from build123d import *

# Parameters (mm, degrees)
EXTRUDE_1_DEPTH     = 15
CUT_EXTRUDE_1_DEPTH = 15
FILLET_1_R          = 1
SKETCH_3_W          = 11.5
SKETCH_3_H          = 1.4
CUT_EXTRUDE_2_DEPTH = 10


with BuildPart() as part:
    # 草图1 → 凸台-拉伸1 (new body)
    with BuildSketch(Plane(origin=(0, 0, 0), x_dir=(1, 0, 0), z_dir=(0, 1, 0))):
        Polygon((-5.74789916, 13.058823529), (2.25210084, 13.058823529), (2.25210084, -11.941176471), (-2.74789916, -11.941176471), (-2.74789916, 4.558823529), (-5.74789916, 4.558823529), align=None)
    extrude(amount=EXTRUDE_1_DEPTH)

    # 草图2 → 切除-拉伸1 (cut)
    with BuildSketch(Plane.ZY.offset(5.74789916)):
        with BuildLine():
            ThreePointArc((-6.483823529, 7.5), (-8.058823529, 9.075), (-9.633823529, 7.5))
            Line((-9.633823529, 7.5), (-6.483823529, 7.5))
        make_face()
        with BuildLine():
            Line((-6.483823529, 7.5), (-9.633823529, 7.5))
            ThreePointArc((-9.633823529, 7.5), (-8.058823529, 5.925), (-6.483823529, 7.5))
        make_face()
    extrude(amount=-CUT_EXTRUDE_1_DEPTH, mode=Mode.SUBTRACT)

    # 圆角1
    fillet_1_edges = [part.edges().sort_by_distance(p)[0] for p in [
        (-2.74789916, 7.5, -4.558823529),
    ]]
    fillet(fillet_1_edges, radius=FILLET_1_R)

    # 草图3 → 切除-拉伸2 (cut)
    with BuildSketch(Plane.ZY.offset(2.74789916)):
        with Locations((1.191176471, 8.2)):
            Rectangle(SKETCH_3_W, SKETCH_3_H)
        with Locations((1.191176471, 6.8)):
            Rectangle(SKETCH_3_W, SKETCH_3_H)
    extrude(amount=-CUT_EXTRUDE_2_DEPTH, mode=Mode.SUBTRACT)


solid = part.part
Model file for the job. Use its own axes, mm. A direction names the side the tool comes from. Give positions to 0.01 mm unless a question says otherwise; leave off trailing zeros. Order: outer loops, then holes, each group sorted by start corner. A loop starts at its lowest first (then second) coordinate and runs counter-clockwise, first axis right, second up. Notation, with made-up numbers: (-33.75, 31) -> (17.25, 31) arc R25 cw to (17.25, 49) -> close; hole circle Ø1 at (24, 82.5). An arc over 180 degrees is marked (long way). Use CSV: the item, a comma, the result in double quotes.
1. Band-saw the part on B-B, the plane y = 7.5. Give the cut face in (x, z), then the cut area to 3 significant figures.
Outcome:
outline,"(-5.75, -13.06) -> (2.25, -13.06) -> (2.25, -9.63) -> (-5.75, -9.63) -> close; (-5.75, -6.48) -> (2.25, -6.48) -> (2.25, -4.56) -> (-2.75, -4.56) -> (-2.75, -3.56) arc R1 cw to (-3.75, -4.56) -> (-5.75, -4.56) -> close; (-2.75, 6.94) -> (2.25, 6.94) -> (2.25, 11.94) -> (-2.75, 11.94) -> close"
area,"68.0 mm²"
2. Band-saw the part on C-C, the plane x = -2. Give the cut face in (y, z) (3 decimals).
Outcome:
outline,"(0, -13.059) -> (15, -13.059) -> (15, 11.941) -> (0, 11.941) -> close; hole circle Ø3.15 at (7.5, -8.059); hole (6.1, -4.559) -> (8.9, -4.559) -> (8.9, 6.941) -> (6.1, 6.941) -> close"
3. Band-saw the part on A-A, the plane z = 5.75. Give the cut face in (x, y), then the cut area to 3 significant figures.
Outcome:
outline,"(-2.75, 0) -> (2.25, 0) -> (2.25, 6.1) -> (-2.75, 6.1) -> close; (-2.75, 8.9) -> (2.25, 8.9) -> (2.25, 15) -> (-2.75, 15) -> close"
area,"61.0 mm²"
4. 3-axis set-ups, long thin cutter, end or side, ignore diameter. For faces 4 (the flat face through (0, 8, -4.559)), 5 (the flat face through (-2.748, 9.1, 4.3)), 6 (the flat face through (0, 7, 6.941)): which of +Z, -Z, +X, -X, +Y, -Y reach the whole face in a straight line?
Outcome:
face 4,"+X"
face 5,"+Z, -X, +Y, -Y"
face 6,"+X, -X"
5. Drop flat-ended pins along their axis: pin 1 (1.5 mm diameter, centred on y = 10.5, z = 0, fed in from -X); pin 2 (0.6 mm diameter, centred on x = -4.5, y = 8, fed in from +Z); pin 3 (2.5 mm diameter, centred on y = 7.5, z = -8.06, fed in from +X). Give the stop position or say it passes through.
Outcome:
pin 1,"x = -2.75"
pin 2,"z = -4.56"
pin 3,"through"
6. Mould opens along Y. For faces 1 (the flat face through (-5.748, 7, -10)), 2 (the flat face through (-2.748, 7.5, -4.2)), 3 (the flat face through (-1, 15, -1)) say: +Y half, -Y half, draft (parallel to the pull), parting line (faces both ways), or undercut.
Outcome:
face 1,"draft"
face 2,"undercut"
face 3,"+Y half"
7. Band-saw the part on D-D, the plane y = 11.75. Give the cut face in (x, z), then the cut area to 3 significant figures.
Outcome:
outline,"(-5.75, -13.06) -> (2.25, -13.06) -> (2.25, 11.94) -> (-2.75, 11.94) -> (-2.75, -3.56) arc R1 cw to (-3.75, -4.56) -> (-5.75, -4.56) -> close"
area,"151 mm²"
8. Drill centre lines: line 1 along Z through (x, y) = (-1.5, 7.5); line 2 along Z through (x, y) = (-2.5, 6.5); line 3 along Y through (x, z) = (1, 0). Where is each one in solid material? Low to high. Write a range as from..to.
Outcome:
line 1,"-13.06..-9.63, -6.48..-4.56, 6.94..11.94"
line 2,"-13.06..-9.28, -6.84..-4.56, 6.94..11.94"
line 3,"0..6.1, 8.9..15"
